Geometry check sheet. Reference: the model listing, model coordinates, mm. A direction names the side the tool comes from. Coordinates: 2 decimals unless noted, no trailing zeros. Loops run counter-clockwise (first coordinate to the right, second up) from the corner with the lowest first, then second, coordinate; pieces in that order, holes last. Notation, with made-up numbers: (34.25, 6) - (46.25, 6) arc R9 ccw to (46.25, 23) - close; hole circle Ø8 at (7, -32). An arc over 180 degrees is marked (long way). Write item = value, one per line. Start each with the question number.
from build123d import *

# Parameters (mm, degrees)
BOSS_EXTRUDE1_DEPTH = 117.5
SKETCH3_R           = 1.75
CUT_EXTRUDE2_DEPTH  = 121.541486634
CHAMFER1_SIZE       = 3


with BuildPart() as part:
    # Sketch1 → Boss-Extrude1 (new, symmetric)
    with BuildSketch(Plane.XY):
        Polygon((0, 0), (20, 0), (20, 2), (2, 2), (2, 20), (0, 20), align=None)
    extrude(amount=BOSS_EXTRUDE1_DEPTH, both=True)

    # Cut-Extrude1 cone 1 section (through the dimple's axis) → Cut-Extrude1 (revolve, cut)
    with BuildSketch(Plane(origin=(10, 2, -107.5), x_dir=(0, 0, 1), z_dir=(1, 0, 0))):
        Polygon((0, 0), (3.5, 0), (0, 3.5), align=None)
    revolve(axis=Axis((10, 2, -107.5), (0, -1, 0)), mode=Mode.SUBTRACT)

    # Cut-Extrude1 cone 2 section (through the dimple's axis) → Cut-Extrude1 cone 2 (revolve, cut)
    with BuildSketch(Plane(origin=(10, 2, 107.5), x_dir=(0, 0, 1), z_dir=(1, 0, 0))):
        Polygon((0, 0), (3.5, 0), (0, 3.5), align=None)
    revolve(axis=Axis((10, 2, 107.5), (0, -1, 0)), mode=Mode.SUBTRACT)

    # Sketch3 → Cut-Extrude2 (cut, through all)
    with BuildSketch(Plane(origin=(0, 2, 0), x_dir=(1, 0, 0), z_dir=(0, 1, 0))):
        with Locations(Location((10, -107.5, 0), (0, 0, 180))):
            Circle(SKETCH3_R)
        with Locations(Location((10, 107.5, 0), (0, 0, 180))):
            Circle(SKETCH3_R)
    extrude(amount=-CUT_EXTRUDE2_DEPTH, mode=Mode.SUBTRACT)

    # Chamfer1
    chamfer1_edges = [part.edges().sort_by_distance(p)[0] for p in [
        (20, 1, 117.5),
        (1, 20, 117.5),
        (1, 20, -117.5),
        (20, 1, -117.5),
    ]]
    chamfer(chamfer1_edges, length=CHAMFER1_SIZE)


solid = part.part
(1) Depth check by flat-ended pin: pin 1 (3 mm diameter, centred on x = 17, z = -56.5, fed in from +Y); pin 2 (10 mm diameter, centred on y = 13.5, z = -83, fed in from +X). Enter the tip coordinate at first touch or a pass-through.
(2) Sectioned sample at B-B on y = 7.75. Enter the section's corners in (x, z).
(3) Sectioned sample at A-A on z = 101.5. Enter the section's corners in (x, y), plus the area to 3 significant figures.
(4) Tool access check on faces 1 (the face through (2, 11, 2)), 2 (the face through (4.7, 1.6, -117.5)). Record the directions out of +Z, -Z, +X, -X, +Y, -Y that give a thin tool (end or side, any length) a straight path to the whole face; none if there is none.
(5) Scan lines: line 1 (Z direction, x = 10, y = 0.1); line 2 (X direction, y = 0.2, z = -107.5). Record each from-to range of solid material in increasing order.
Working result:
q1.pin_1 = 2
q1.pin_2 = 2
q2.outline = (0, -117.5) - (2, -117.5) - (2, 117.5) - (0, 117.5) - close
q3.outline = (0, 0) - (20, 0) - (20, 2) - (2, 2) - (2, 20) - (0, 20) - close
q3.area = 76.0 mm2
q4.face_1 = +Z, -Z, +X, +Y
q4.face_2 = -Z, +X, -X, +Y, -Y
q5.line_1 = -117.5 to -109.25, -105.75 to 105.75, 109.25 to 117.5
q5.line_2 = 0 to 8.25, 11.75 to 20
